from build123d import *

# Parameters (mm, degrees)
SKETCH2_W           = 160
SKETCH2_H           = 80
BOSS_EXTRUDE1_DEPTH = 30
CUT_EXTRUDE1_DEPTH  = 168.630546142
SKETCH4_R           = 7.5
CUT_EXTRUDE2_DEPTH  = 95.339811321
BOSS_EXTRUDE2_START = -40
SKETCH5_R           = 12.5
BOSS_EXTRUDE2_DEPTH = 20
FILLET1_R           = 2


with BuildPart() as part:
    # Sketch2 → Boss-Extrude1 (new body)
    with BuildSketch(Plane(origin=(0, 0, 0), x_dir=(1, 0, 0), z_dir=(0, 1, 0))):
        Rectangle(SKETCH2_W, SKETCH2_H)
    extrude(amount=BOSS_EXTRUDE1_DEPTH)

    # Sketch3 → Cut-Extrude1 (cut, through all)
    with BuildSketch(Plane(origin=(80, 0, 0), x_dir=(0, 0, -1), z_dir=(1, 0, 0))):
        Polygon((-25, 15), (-16.339745962, 0), (16.339745962, 0), (25, 15), align=None)
    extrude(amount=-CUT_EXTRUDE1_DEPTH, mode=Mode.SUBTRACT)

    # Sketch4 → Cut-Extrude2 (cut, through all)
    with BuildSketch(Plane(origin=(0, 30, 0), x_dir=(1, 0, 0), z_dir=(0, 1, 0))):
        with Locations(Location((60, 0, 0), (0, 0, 270))):
            Circle(SKETCH4_R)
    cut_extrude2 = extrude(amount=-CUT_EXTRUDE2_DEPTH, mode=Mode.SUBTRACT)

    # Sketch5 → Boss-Extrude2 (add)
    with BuildSketch(Plane(origin=(80, 0, 0), x_dir=(0, 0, -1), z_dir=(1, 0, 0)).offset(BOSS_EXTRUDE2_START)):
        with BuildLine():
            ThreePointArc((25, 55), (0, 80), (-25, 55))
            Line((-25, 55), (-25, 30))
            Line((-25, 30), (25, 30))
            Line((25, 30), (25, 55))
        make_face()
        with Locations((0, 55)):
            Circle(SKETCH5_R, mode=Mode.SUBTRACT)
    boss_extrude2 = extrude(amount=-BOSS_EXTRUDE2_DEPTH)

    # Mirror1: Cut-Extrude2, Boss-Extrude2 across plane
    add(cut_extrude2.mirror(Plane(origin=(0, 0, 0), x_dir=(0, 0, 1), z_dir=(1, 0, 0))), mode=Mode.SUBTRACT)
    add(boss_extrude2.mirror(Plane(origin=(0, 0, 0), x_dir=(0, 0, 1), z_dir=(1, 0, 0))))

    # Fillet1
    fillet1_edges = [part.edges().sort_by_distance(p)[0] for p in [
        (30, 30, -25),
        (30, 30, 25),
        (-30, 30, 25),
        (-30, 30, -25),
    ]]
    fillet(fillet1_edges, radius=FILLET1_R)


solid = part.part
Could you check a few things on this model? Use its own coordinates, in mm. A direction names the side the tool comes from. Coordinates: 2 decimals unless noted, no trailing zeros. Order: outer loops, then holes, each group sorted by start corner. A loop starts at its lowest first (then second) coordinate and runs counter-clockwise, first axis right, second up. Notation, with made-up numbers: (-19.75, 74) - (19.25, 74) arc R24 ccw to (19.25, 94) - close; hole circle Ø11 at (49.25, 58). An arc over 180 degrees is marked (long way). Answer in a Markdown table with one row per item. Add a question column.
(1) If we section it at D-D, the plane x = -60: Please give me the cut outline in (y, z), then the cut area to 3 significant figures.
(2) If we section it at B-B, the plane z = 0: Please give me the cut outline in (x, y).
(3) Will these pins go through, and if not, where does the flat tip stop? pin 1 (25 mm diameter, centred on y = 58.5, z = -6.5, fed in from -X); pin 2 (1 mm diameter, centred on x = -21, y = 32.5, fed in from +Z); pin 3 (10 mm diameter, centred on x = -27, y = 43, fed in from -Z); pin 4 (12 mm diameter, centred on x = 31.5, z = 13.5, fed in from -Y).
(4) I need wall thicknesses on L1, parallel to X at y = 22, z = 0; L2, parallel to Y at x = -27, z = 0; L3, parallel to X at y = 46.5, z = -11. Which ranges of each line are inside material? Lowest first, please.
(5) If we mould it in two halves opening along Y, with no side actions, what happens to faces 5 (the face through (1.12, 7.4, -20.61)), 6 (the face through (-67.436, 22.605, -0.976)), 7 (the face through (-1, 0, -28))? For each: released by +Y, released by -Y, zero draft, split by the parting line, or undercut.
(6) If we section it at A-A, the plane x = -30.5: Please give me the cut outline in (y, z).
(7) On a 3-axis mill with a long thin cutter (end or side, diameter ignored), from which of +Z, -Z, +X, -X, +Y, -Y can I reach the whole of each face in a straight line? I mean faces 1 (the face through (40, 50, -12)), 2 (the face through (-30, 44, 25)), 3 (the face through (-30, 43, -25)), 4 (the face through (20, 50, -12)). Say none if no direction works.
(8) If we section it at C-C, the plane y = 12: Please give me the cut outline in (x, z).
Results are:
| question | item | result |
|---|---|---|
| 1 | outline | (0, -40) - (30, -40) - (30, -7.5) - (15, -7.5) - (15, -25) - (0, -16.34) - close; (0, 16.34) - (15, 25) - (15, 7.5) - (30, 7.5) - (30, 40) - (0, 40) - close |
| 1 | area | 1,550 mm2 |
| 2 | outline | (-80, 15) - (-67.5, 15) - (-67.5, 30) - (-80, 30) - close; (-52.5, 15) - (52.5, 15) - (52.5, 30) - (40, 30) - (40, 42.5) - (20, 42.5) - (20, 30) - (-20, 30) - (-20, 42.5) - (-40, 42.5) - (-40, 30) - (-52.5, 30) - close; (-40, 67.5) - (-20, 67.5) - (-20, 80) - (-40, 80) - close; (20, 67.5) - (40, 67.5) - (40, 80) - (20, 80) - close; (67.5, 15) - (80, 15) - (80, 30) - (67.5, 30) - close |
| 3 | pin 1 | stops at x = -40 |
| 3 | pin 2 | stops at z = 25 |
| 3 | pin 3 | stops at z = -25 |
| 3 | pin 4 | stops at y = 0 |
| 4 | L1 | x = -80 to -67.5, -52.5 to 52.5, 67.5 to 80 |
| 4 | L2 | y = 15 to 42.5, 67.5 to 80 |
| 4 | L3 | x = -40 to -20, 20 to 40 |
| 5 | face 5 | undercut |
| 5 | face 6 | zero draft |
| 5 | face 7 | released by -Y |
| 6 | outline | (0, -40) - (30, -40) - (30, -27) arc R2 cw to (32, -25) - (55, -25) arc R25 ccw to (55, 25) - (32, 25) arc R2 cw to (30, 27) - (30, 40) - (0, 40) - (0, 16.34) - (15, 25) - (15, -25) - (0, -16.34) - close; hole circle Ø25 at (55, 0) |
| 7 | face 1 | +Z, -Z, +X, +Y |
| 7 | face 2 | +Z, +X, -X, +Y |
| 7 | face 3 | -Z, +X, -X, +Y |
| 7 | face 4 | +Z, -Z, +Y |
| 8 | outline | (-80, -40) - (80, -40) - (80, -23.27) - (-80, -23.27) - close; (-80, 23.27) - (80, 23.27) - (80, 40) - (-80, 40) - close |
